Here's how the part is built. I have some questions about the finished solid (model axes, mm). Face numbers are marked on the shaded views. Round coordinates to 2 decimals unless told otherwise and drop trailing zeros. Order: outer loops, then holes, each group sorted by start corner. A loop starts at its lowest first (then second) coordinate and runs counter-clockwise, first axis right, second up. Notation, with made-up numbers: (-11, 19.5) -> (-5, 19.5) arc R26 cw to (-5, 49.5) -> close; hole circle Ø10 at (76, 19.25). An arc over 180 degrees is marked (long way). One line per item, written item: value.
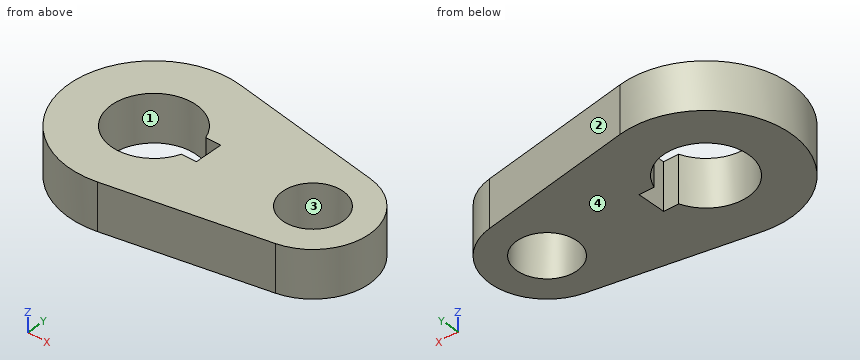
```python
from build123d import *

# Parameters (mm, degrees)
F0_R     = 10.16
F1_DEPTH = 15.7734


with BuildPart() as f1:
    # F0 (on Top) → F1 (new body)
    with BuildSketch(Plane.XY):
        with BuildLine():
            ThreePointArc((5.042647, 28.126541), (-28.575, 0), (5.042647, -28.126541))
            ThreePointArc((5.042647, -28.126541), (21.916025, -18.336262), (28.575, 0))
            ThreePointArc((28.575, 0), (21.916025, 18.336262), (5.042647, 28.126541))
        make_face()
        with BuildLine():
            ThreePointArc((13.447765, -4.826), (-14.2875, 0), (13.447765, 4.826))
            Line((13.447765, 4.826), (18.5293, 4.826))
            Line((18.5293, 4.826), (18.5293, -4.826))
            Line((18.5293, -4.826), (13.447765, -4.826))
        make_face(mode=Mode.SUBTRACT)
        with BuildLine():
            Line((5.042647, -28.126541), (57.336765, -18.751028))
            ThreePointArc((57.336765, -18.751028), (73.025, 0), (57.336765, 18.751028))
            Line((57.336765, 18.751028), (5.042647, 28.126541))
            ThreePointArc((5.042647, 28.126541), (21.916025, 18.336262), (28.575, 0))
            ThreePointArc((28.575, 0), (21.916025, -18.336262), (5.042647, -28.126541))
        make_face()
        with Locations((53.975, 0)):
            Circle(F0_R, mode=Mode.SUBTRACT)
    extrude(amount=F1_DEPTH)


solid = f1.part
```
Q1. For P1, Ø2.5, axis at x = 16.5, z = 7.5, coming from the -Y side; P2, Ø1, axis at x = 60.5, z = 2, coming from the -Y side; P3, Ø2, axis at y = -3.5, z = 9, coming from the -X side; P4, Ø6, axis at x = -2, z = 13, coming from the -Y side (3 decimals), each with a flat end and sliding along its axis, tell me the tip position at first contact or that it passes through.
Answers:
P1: y = -26.3
P2: y = -18.07
P3: x = -28.47
P4: y = -28.575
Q2. I want a section at B-B on z = 14. Give the number of separate pieces and of enclosed holes in the cut face, then the cut area to 3 significant figures.
Answers:
separate pieces: 1
enclosed holes: 2
area: 3,450 mm2
Q3. I want a section at C-C on x = 0. Write out the boundary of the cut face in (y, z) (1 decimal).
Answers:
outline: (-28.6, 0) -> (-14.3, 0) -> (-14.3, 15.8) -> (-28.6, 15.8) -> close; (14.3, 0) -> (28.6, 0) -> (28.6, 15.8) -> (14.3, 15.8) -> close
Q4. I want a section at D-D on y = -12. Write out the boundary of the cut face in (x, z), then the cut area to 3 significant figures.
Answers:
outline: (-25.93, 0) -> (-7.75, 0) -> (-7.75, 15.77) -> (-25.93, 15.77) -> close; (7.75, 0) -> (68.77, 0) -> (68.77, 15.77) -> (7.75, 15.77) -> close
area: 1,250 mm2
Q5. I want a section at A-A on y = 0. Write out the boundary of the cut face in (x, z) (1 decimal).
Answers:
outline: (-28.6, 0) -> (-14.3, 0) -> (-14.3, 15.8) -> (-28.6, 15.8) -> close; (18.5, 0) -> (43.8, 0) -> (43.8, 15.8) -> (18.5, 15.8) -> close; (64.1, 0) -> (73, 0) -> (73, 15.8) -> (64.1, 15.8) -> close
Q6. If we mould it in two halves opening along X, with no side actions, what happens to the marked faces 1, 2, 3 and 4? For each: pulls with the +X half, pulls with the -X half, needs draft (parallel to the pull), parting line crosses it, or undercut.
Answers:
face 1: undercut
face 2: pulls with the +X half
face 3: undercut
face 4: needs draft
Q7. I need wall thicknesses on line 1 along Y through (x, z) = (0, 3) (1 decimal); line 2 along X through (y, z) = (-0.5, 1); line 3 along X through (y, z) = (-4, 7.25). Which ranges of each line are inside material? Lowest first, please.
Answers:
line 1: -28.6 to -14.3, 14.3 to 28.6
line 2: -28.57 to -14.28, 18.53 to 43.83, 64.12 to 73.02
line 3: -28.29 to -13.72, 18.53 to 44.64, 63.31 to 72.6
